Source: three-view drawing plus pictorial views. Frame: mm from the lowest corner of the part. A direction names the side the tool comes from. Coordinates: 2 decimals unless noted, no trailing zeros. Write each loop counter-clockwise with the first axis right and the second up, starting at its lowest first coordinate (ties: lowest second). Pieces come first, ordered by that corner, then holes.
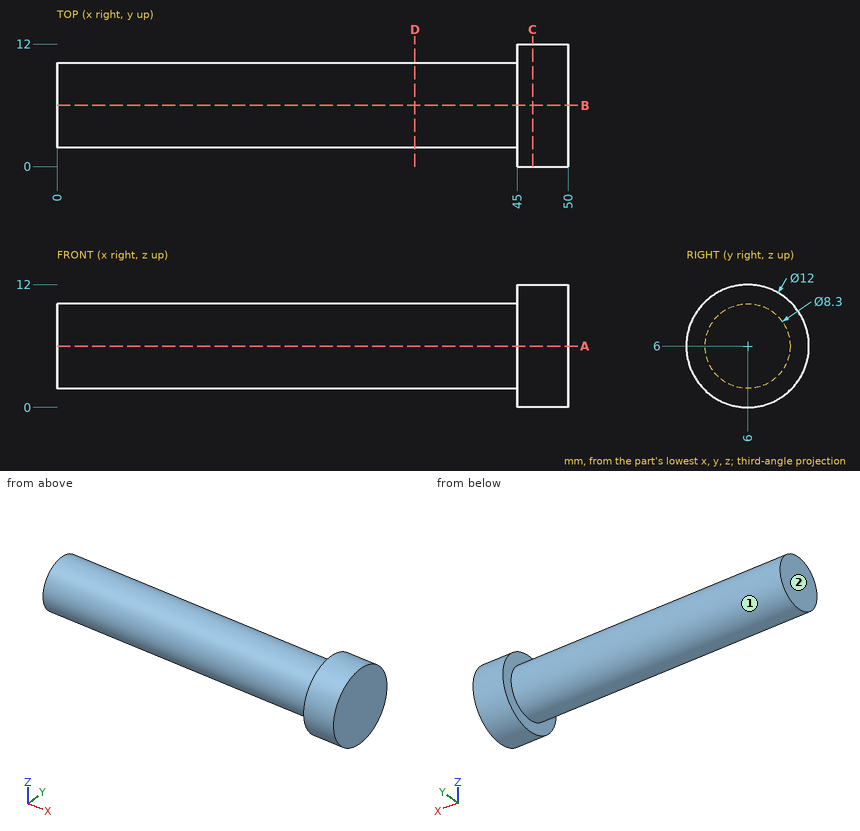
Item 1: Material intervals for line 1 (Z direction, x = 7.5, y = 6.25); line 2 (X direction, y = 3.5, z = 2); line 3 (Z direction, x = 28, y = 8), sorted ascending.
Item 2: Access query for the marked faces 1 and 2. Directions: +Z, -Z, +X, -X, +Y, -Y. A direction counts if a zero-diameter tool reaches every point of the face in a straight line with its end or side. Return the directions, or none.
Item 3: Pin query (flat end, axial travel): pin 1 Ø4 at (x, y) = (34.5, 7) entering from +Z. Return the tip coordinate at first contact, or that it passes through.
Item 4: Section query A-A, the plane z = 6. Return loops of the section in (x, y), then the cut area to 4 significant figures.
Item 5: Section query C-C, the plane x = 46.5. Return loops of the section in (y, z), then the cut area to 3 significant figures.
Item 6: Section query D-D, the plane x = 35. Return loops of the section in (y, z).
The answers:
1. line 1: z = 1.86 to 10.14
1. line 2: x = 45 to 50
1. line 3: z = 2.36 to 9.64
2. face 1: -X
2. face 2: +Z, -Z, -X, +Y, -Y
3. pin 1: stops at z = 10.15
4. outline: (0, 1.85) - (45, 1.85) - (45, 0) - (50, 0) - (50, 12) - (45, 12) - (45, 10.15) - (0, 10.15) - close
4. area: 433.5 mm2
5. outline: circle Ø12 at (6, 6)
5. area: 113 mm2
6. outline: circle Ø8.3 at (6, 6)
